Read the model definition and answer for the solid it produces. Units are mm, in the model's axes. Face numbers are marked on the shaded views. A direction names the side the tool comes from. Round coordinates to 2 decimals unless told otherwise and drop trailing zeros. Order: outer loops, then holes, each group sorted by start corner. A loop starts at its lowest first (then second) coordinate and runs counter-clockwise, first axis right, second up. Notation, with made-up numbers: (11.5, 12.5) - (28.5, 12.5) arc R29 cw to (28.5, 45.5) - close; hole circle Ø1 at (66.25, 38.25). An arc over 180 degrees is marked (long way). Put each result on its own line as item: value. Start each with the question number.
Q1. Each of these flat-tipped pins is pushed along its axis until it touches: pin 1 Ø1.6 at (y, z) = (1.5, -31) entering from +X; pin 2 Ø1 at (y, z) = (16, -32) entering from +X; pin 3 Ø4 at (x, z) = (17, -31.5) entering from -Y. Where does it stop, or does it pass through?
Q2. Section C-C on x = 5.75 is taken. Give the vertices of the cut face in (y, z).
Q3. Section B-B on z = -32.5 is taken. Give the vertices of the cut face in (x, y), then the cut area to 3 significant figures.
Q4. For a pull along X with two mould halves and no side action, classify the marked faces 3, 4 and 5 as pulls with the +X half, pulls with the -X half, needs draft (parallel to the pull), parting line crosses it, or undercut.
Q5. Which of the six approach directions +Z, -Z, +X, -X, +Y, -Y give full straight-line access (tool end or side, diameter ignored) to the marked faces 1 and 2?
Q6. Find the intervals of material crossed by line 1 along X through (y, z) = (5.5, -34); line 2 along Y through (x, z) = (22.5, -18); line 3 along X through (y, z) = (11.5, -3), in increasing order. Write a range as from..to.
Q7. Section D-D on z = -18 is taken. Give the vertices of the cut face in (x, y), then the cut area to 3 significant figures.
Q8. Section A-A on x = 14.25 is taken. Give the vertices of the cut face in (y, z), then the cut area to 3 significant figures.
from build123d import *

# Parameters (mm, degrees)
F0_W      = 29
F0_H      = 16.5
F1_DEPTH  = 38.5
F2_T      = -2
F3_DEPTH  = 2.25
F4_SIZE   = 2
F5_SIZE   = 2
F6_SIZE   = 0.99999
F8_DEPTH  = 16.501
F9_W      = 7.54
F9_H      = 7.25
F9_R      = 1.1
F10_DEPTH = 4.35


# Not quite as in the source:
# - a fillet or chamfer is up to 0.001 mm smaller than in the source, because OpenCascade refuses the exact size


with BuildPart() as f1:
    # F0 (on Top) → F1 (new body)
    with BuildSketch(Plane.XY):
        with Locations((14.5, 8.25)):
            Rectangle(F0_W, F0_H)
    extrude(amount=-F1_DEPTH)

    # F2
    f2_openings = [f1.faces().sort_by_distance(p)[0] for p in [
        (14.5, 8.25, 0),
    ]]
    offset(amount=F2_T, openings=f2_openings)

    # F3 (add): a face of the model
    f3_faces = [f1.faces().sort_by_distance(p)[0] for p in [
        (14.5, 8.25, -36.5),
    ]]
    extrude(f3_faces, amount=F3_DEPTH)

    # F4
    f4_edges = [f1.edges().sort_by_distance(p)[0] for p in [
        (29, 0, -19.25),
        (0, 0, -19.25),
        (0, 16.5, -19.25),
        (29, 16.5, -19.25),
    ]]
    chamfer(f4_edges, length=F4_SIZE)

    # F5
    f5_edges = [f1.edges().sort_by_distance(p)[0] for p in [
        (0, 8.25, -38.5),
        (1, 15.5, -38.5),
        (1, 1, -38.5),
        (14.5, 16.5, -38.5),
        (14.5, 0, -38.5),
        (28, 15.5, -38.5),
        (28, 1, -38.5),
        (29, 8.25, -38.5),
    ]]
    chamfer(f5_edges, length=F5_SIZE)

    # F6 (size 1 in the source; OpenCascade refuses exactly that, so slightly less here)
    f6_edges = [f1.edges().sort_by_distance(p)[0] for p in [
        (0, 8.25, 0),
        (14.5, 16.5, 0),
        (29, 8.25, 0),
        (14.5, 0, 0),
    ]]
    chamfer(f6_edges, length=F6_SIZE)

    # F7 (on face) → F8 (cut, through all)
    with BuildSketch(Plane.XZ):
        Polygon((23.536, -33.56), (23.536, -29.836), (17.365, -25.666), (12.635, -25.666), (6.464, -29.836), (6.464, -33.56), align=None)
    extrude(amount=-F8_DEPTH, mode=Mode.SUBTRACT)

    # F9 (on face) → F10 (join)
    with BuildSketch(Plane(origin=(0, 0, 0), x_dir=(0, -1, 0), z_dir=(-1, 0, 0))):
        with Locations((-8.25, -30.625)):
            Rectangle(F9_W, F9_H)
        with Locations((-8.25, -29.5)):
            Circle(F9_R, mode=Mode.SUBTRACT)
        with Locations((-8.25, -29.5)):
            Circle(F9_R)
    extrude(amount=-F10_DEPTH)


solid = f1.part
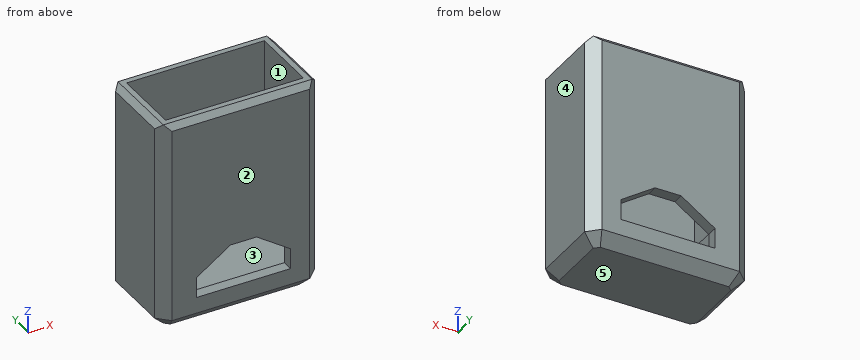
Findings:
1. pin 1: x = 29
1. pin 2: x = 28
1. pin 3: through
2. outline: (0, -36.5) - (2, -38.5) - (14.5, -38.5) - (16.5, -36.5) - (16.5, -1) - (15.5, 0) - (14.5, 0) - (14.5, -34.25) - (2, -34.25) - (2, 0) - (1, 0) - (0, -1) - close
3. outline: (0, 2) - (2, 0) - (6.46, 0) - (6.46, 2) - (2, 2) - (2, 4.48) - (4.35, 4.48) - (4.35, 12.02) - (2, 12.02) - (2, 14.5) - (6.46, 14.5) - (6.46, 16.5) - (2, 16.5) - (0, 14.5) - close; (23.54, 0) - (27, 0) - (29, 2) - (29, 14.5) - (27, 16.5) - (23.54, 16.5) - (23.54, 14.5) - (27, 14.5) - (27, 2) - (23.54, 2) - close
3. area: 107 mm2
4. face 3: undercut
4. face 4: pulls with the +X half
4. face 5: needs draft
5. face 1: +Z
5. face 2: +Z, -Z, +X, -X, -Y
6. line 1: 0..4.35, 27..29
6. line 2: 0..2, 14.5..16.5
6. line 3: 0..2, 27..29
7. outline: (0, 2) - (2, 0) - (27, 0) - (29, 2) - (29, 14.5) - (27, 16.5) - (2, 16.5) - (0, 14.5) - close; hole (2, 2) - (27, 2) - (27, 14.5) - (2, 14.5) - close
7. area: 158 mm2
8. outline: (0, -36.5) - (2, -38.5) - (14.5, -38.5) - (16.5, -36.5) - (16.5, -33.56) - (14.5, -33.56) - (14.5, -34.25) - (2, -34.25) - (2, -33.56) - (0, -33.56) - close; (0, -25.67) - (2, -25.67) - (2, 0) - (1, 0) - (0, -1) - close; (14.5, -25.67) - (16.5, -25.67) - (16.5, -1) - (15.5, 0) - (14.5, 0) - close
8. area: 171 mm2
